Answer from the drawing. Dimensions are ordinates in mm from the lowest x, y and z of the part. Give positions to 0.01 mm unless a question says otherwise; leave off trailing zeros. Loops run counter-clockwise (first coordinate to the right, second up) from the corner with the lowest first, then second, coordinate; pieces in that order, holes last. Notation, with made-up numbers: (16, 81) - (40, 81) arc R19 ccw to (40, 90) - close; hole circle Ø5 at (51.25, -23.75). An arc over 180 degrees is marked (long way). One line per question, with ' | ' between items. Start each with the question number.
1. For a pull along Y with two mould halves and no side action, classify the marked faces 1, 2, 3 and 4 as released by +Y, released by -Y, zero draft, split by the parting line, or undercut.
2. This flat-tipped pin is pushed along its axis until it touches: pin 1 (13.5 mm diameter, centred on x = 25.4, y = 25.4, fed in from +Z). Where does it stop, or does it pass through?
3. Find the intervals of material crossed by line 1 (Y direction, x = 25, z = 121); line 2 (X direction, y = 23, z = 103), in increasing order.
4. Section A-A (z = 126.5) is taken. Determine the outline of the cut face in (x, y) (1 decimal).
5. Section B-B (z = 88) is taken. Determine the outline of the cut face in (x, y), plus the area to 3 significant figures.
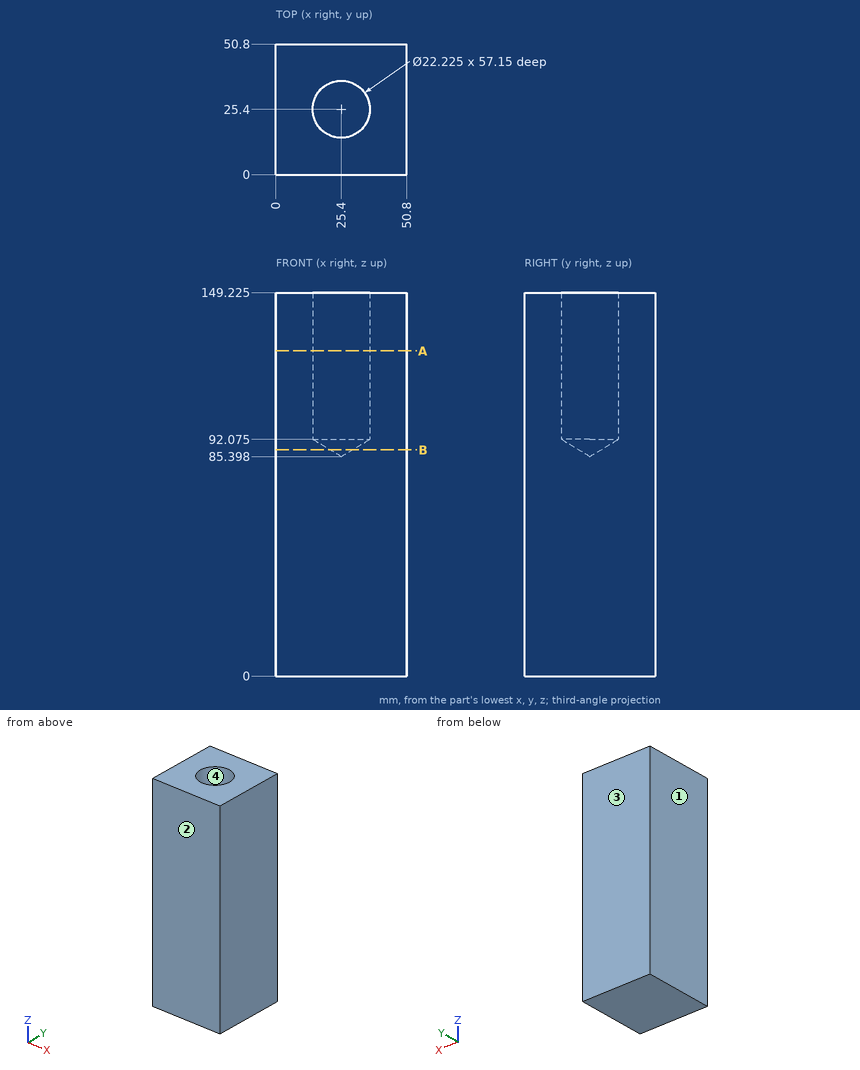
Conclusion:
1) face 1: zero draft | face 2: released by -Y | face 3: released by +Y | face 4: undercut
2) pin 1: z = 89.45
3) line 1: 0 to 14.29, 36.51 to 50.8 | line 2: 0 to 14.55, 36.25 to 50.8
4) outline: (0, 0) - (50.8, 0) - (50.8, 50.8) - (0, 50.8) - close; hole circle Ø22.2 at (25.4, 25.4)
5) outline: (0, 0) - (50.8, 0) - (50.8, 50.8) - (0, 50.8) - close; hole circle Ø8.66 at (25.4, 25.4) | area: 2,520 mm²
